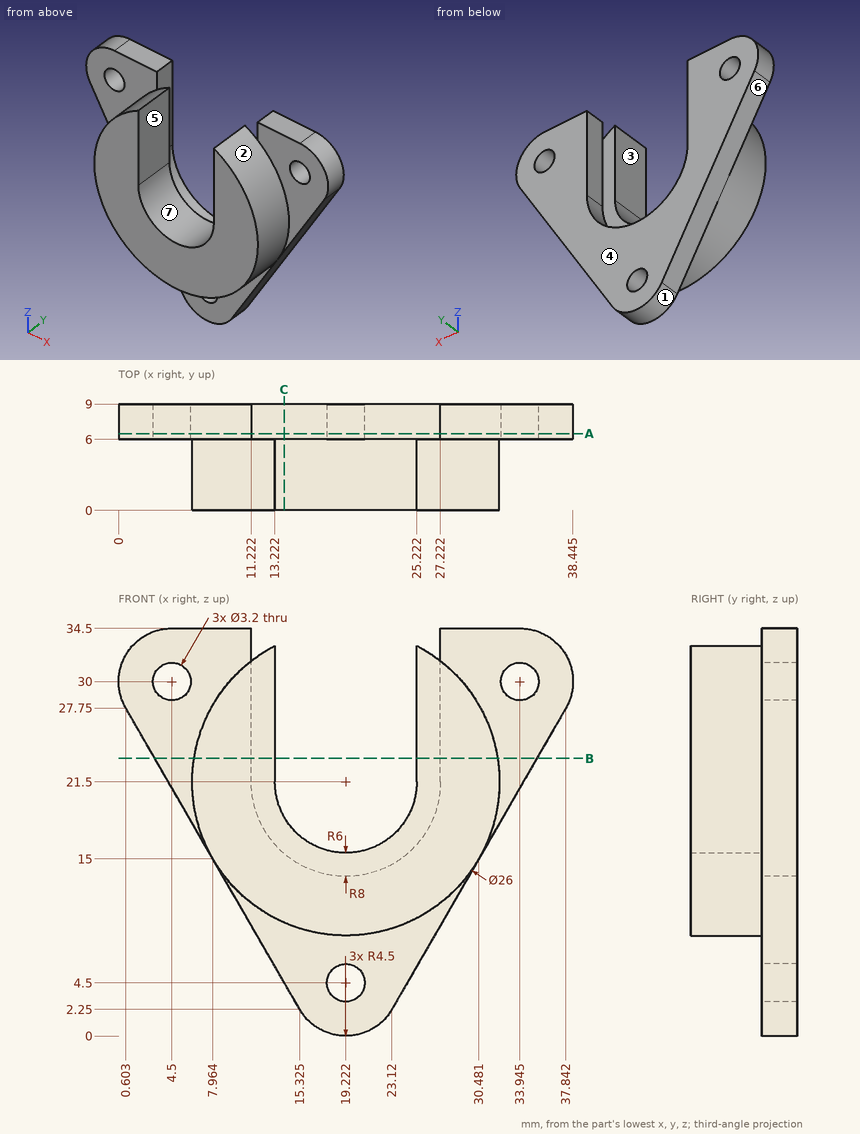
Job drawing, mm, ordinate dimensions from the low corner. One solid piece. A direction names the side the tool comes from. Coordinates: 2 decimals unless noted, no trailing zeros. Order: outer loops, then holes, each group sorted by start corner. A loop starts at its lowest first (then second) coordinate and runs counter-clockwise, first axis right, second up. Notation, with made-up numbers: (62.25, 45.5) - (114.25, 45.5) arc R27 cw to (114.25, 78.5) - close; hole circle Ø4 at (23, 10.25). An arc over 180 degrees is marked (long way). Return JSON: item names as keys, results as strings. Group by question number.
1) Probe line 1 (X direction, y = 8.15, z = 30) (1 decimal); line 2 (Y direction, x = 12.5, z = 26.5); line 3 (X direction, y = 1.5, z = 23) (1 decimal). List the from-to ranges inside material, lowest first. Write a range as from..to.
2) Saw through at B-B, the plane z = 23.5. Write the cut outline in (x, y), plus the area to 3 significant figures.
3) Tool access for the marked faces 1, 2 and 3: list every direction of +Z, -Z, +X, -X, +Y, -Y with a clear straight run to the whole face (end or side of a thin tool).
4) Mould opens along X. For the marked faces 4, 5, 6 and 7 say: released by +X, released by -X, zero draft, split by the parting line, or undercut.
5) Saw through at A-A, the plane y = 6.5. Count the separate pieces of the cut face and the enclosed holes in it, plus the area to 3 significant figures.
6) Flat gauge pins, fed straight in: P1, Ø1.9, axis at x = 19.22, z = 4.5, coming from the -Y side; P2, Ø4, axis at y = 6.5, z = 5, coming from the +X side; P3, Ø5, axis at y = 2, z = 27.5, coming from the -X side; P4, Ø2, axis at x = 15.5, y = 4, coming from the +Z side. Where does each tip first touch, or does it go through?
7) Saw through at C-C, the plane x = 14. Write the cut outline in (y, z) (1 decimal).
Values found:
{
 "1": {"line 1": "x = 0..2.9, 6.1..11.2, 27.2..32.3, 35.5..38.4", "line 2": "y = 0..6", "line 3": "x = 6.3..13.2, 25.2..32.1"},
 "2": {"outline": "(3.06, 6) - (6.38, 6) - (6.38, 0) - (13.22, 0) - (13.22, 6) - (11.22, 6) - (11.22, 9) - (3.06, 9) - close; (25.22, 0) - (32.07, 0) - (32.07, 6) - (35.39, 6) - (35.39, 9) - (27.22, 9) - (27.22, 6) - (25.22, 6) - close", "area": "131 mm²"},
 "3": {"face 1": "-Z, +Y, -Y", "face 2": "-Y", "face 3": "+Z, +Y, -Y"},
 "4": {"face 4": "zero draft", "face 5": "undercut", "face 6": "released by -X", "face 7": "undercut"},
 "5": {"separate pieces": "1", "enclosed holes": "3", "area": "504 mm²"},
 "6": {"P1": "passes through", "P2": "stops at x = 25.86", "P3": "stops at x = 6.7", "P4": "stops at z = 17.8"},
 "7": {"outline": "(0, 9.6) - (6, 9.6) - (6, 4.5) - (9, 4.5) - (9, 15.4) - (6, 15.4) - (6, 18.5) - (0, 18.5) - close"}
}
